from build123d import *

# Parameters (mm, degrees)
F1_R     = 9.185
F1_R_2   = 4.425
F2_DEPTH = 1
F5_SIZE  = 0.4
F6_SIZE  = 0.2
F7_SIZE  = 0.4
F8_SIZE  = 0.2


with BuildPart() as f2:
    # F1 (on Top) → F2 (new body)
    with BuildSketch(Plane.XY):
        Circle(F1_R)
        Circle(F1_R_2, mode=Mode.SUBTRACT)
    extrude(amount=F2_DEPTH)

    # F5
    f5_edges = [f2.edges().sort_by_distance(p)[0] for p in [
        (-9.185, 0, 0),
    ]]
    chamfer(f5_edges, length=F5_SIZE)

    # F6
    f6_edges = [f2.edges().sort_by_distance(p)[0] for p in [
        (-9.185, 0, 1),
    ]]
    chamfer(f6_edges, length=F6_SIZE)

    # F7
    f7_edges = [f2.edges().sort_by_distance(p)[0] for p in [
        (-4.425, 0, 0),
    ]]
    chamfer(f7_edges, length=F7_SIZE)

    # F8
    f8_edges = [f2.edges().sort_by_distance(p)[0] for p in [
        (-4.425, 0, 1),
    ]]
    chamfer(f8_edges, length=F8_SIZE)


solid = f2.part
Source: CAD feature listing. Evaluate the final solid. Frame: model axes, mm. Give positions to 0.01 mm unless a question says otherwise; leave off trailing zeros. Write each loop counter-clockwise with the first axis right and the second up, starting at its lowest first coordinate (ties: lowest second). Pieces come first, ordered by that corner, then holes. Notation, with made-up numbers: (28, 64) -> (33, 64) arc R29 ccw to (33, 88) -> close; hole circle Ø3 at (-38, 29.25). An arc over 180 degrees is marked (long way). Write item = value, one per line.
Q1. Mould query, pull axis X, two halves, no side actions, for faces 1 (the face through (4, -4, 1)), 2 (the face through (4.22, 1.33, 0.6)), 3 (the face through (-7.29, -5.59, 0.6)). Classes: +X half, -X half, draft (parallel to the pull), parting line (faces both ways), or undercut.
Here are the results:
face_1 = draft
face_2 = undercut
face_3 = parting line
Q2. Cut plane C-C on z = 0.15. Return loops of the section in (x, y) (3 decimals), then the cut area to 3 significant figures.
Here are the results:
outline = circle Ø17.87 at (0, 0); hole circle Ø9.35 at (0, 0)
area = 182 mm²
Q3. Line query: line 1 (Y direction, x = 0, z = 0.5) (3 decimals); line 2 (X direction, y = -1.25, z = 0.85); line 3 (Y direction, x = 2.25, z = 0.5). Output: solid intervals per line, ascending. Write a range as from..to.
Here are the results:
line_1 = -9.185..-4.425, 4.425..9.185
line_2 = -9.05..-4.3, 4.3..9.05
line_3 = -8.91..-3.81, 3.81..8.91
Q4. Cut plane A-A on x = 0. Return loops of the section in (y, z) (3 decimals).
Here are the results:
outline = (-9.185, 0.4) -> (-8.785, 0) -> (-4.825, 0) -> (-4.425, 0.4) -> (-4.425, 0.8) -> (-4.625, 1) -> (-8.985, 1) -> (-9.185, 0.8) -> close; (4.425, 0.4) -> (4.825, 0) -> (8.785, 0) -> (9.185, 0.4) -> (9.185, 0.8) -> (8.985, 1) -> (4.625, 1) -> (4.425, 0.8) -> close
